from build123d import *

# Parameters (mm, degrees)
F0_R     = 9.525
F1_DEPTH = 6.35
F2_R     = 9.525
F3_DEPTH = 12.7


# Not quite as in the source:
# - a length typed as a fraction of an inch, garbled in the dataset ("3 / 203.2 mm" for 3/8 in), is restored


with BuildPart() as f1:
    # F0 (on Top) → F1 (new body)
    with BuildSketch(Plane.XY):
        with BuildLine():
            Line((12.7, 12.7), (0, 12.7))
            ThreePointArc((0, 12.7), (-12.7, 0), (0, -12.7))
            Line((0, -12.7), (12.7, -12.7))
            ThreePointArc((12.7, -12.7), (25.4, 0), (12.7, 12.7))
        make_face()
        Circle(F0_R, mode=Mode.SUBTRACT)
    extrude(amount=F1_DEPTH)

    # F2 (on face) → F3 (join)
    with BuildSketch(Plane(origin=(0, 0, 0), x_dir=(1, 0, 0), z_dir=(0, 0, -1))):
        with BuildLine():
            ThreePointArc((0, -12.7), (8.9802561211, -8.9802561211), (12.7, 0))
            ThreePointArc((12.7, 0), (8.9802561211, 8.9802561211), (0, 12.7))
            ThreePointArc((0, 12.7), (-12.7, 0), (0, -12.7))
        make_face()
        Circle(F2_R, mode=Mode.SUBTRACT)
    extrude(amount=F3_DEPTH)


solid = f1.part
Design review of the part built by this model. Coordinates are the model's own, in mm. A direction names the side the tool comes from. Coordinates: 2 decimals unless noted, no trailing zeros. Write each loop counter-clockwise with the first axis right and the second up, starting at its lowest first coordinate (ties: lowest second). Pieces come first, ordered by that corner, then holes. Notation, with made-up numbers: (-23, 75) - (-19, 75) arc R16 cw to (-19, 105) - close; hole circle Ø6 at (30, -11.5). An arc over 180 degrees is marked (long way). One line per item, written item: value.
1) Add section D-D (x = -0.5). State the section outline as (y, z) points.
Answer sheet:
outline: (-12.69, -12.7) - (-9.51, -12.7) - (-9.51, 6.35) - (-12.69, 6.35) - close; (9.51, -12.7) - (12.69, -12.7) - (12.69, 6.35) - (9.51, 6.35) - close
2) For faces 4 (the face through (10, 0, 6.35)), 5 (the face through (15, 0, 0)), list the 3-axis set-ups (+Z, -Z, +X, -X, +Y, -Y) from which the entire face can be reached by the end or side of a thin tool; tool diameter is ignored.
Answer sheet:
face 4: +Z, +X, -X, +Y, -Y
face 5: -Z, +X
3) Add section B-B (z = -5.75). State the section outline as (x, y) points (3 decimals).
Answer sheet:
outline: circle Ø25.4 at (0, 0); hole circle Ø19.05 at (0, 0)
4) Mouldability with a two-part tool opening along X and no side actions: class faces 1 (the face through (5, -9, -12.7)), 2 (the face through (-7.559, 5.796, -3.042)), 3 (the face through (25.397, -0.279, 3.131)) as +X half, -X half, draft (parallel to the pull), parting line (faces both ways), or undercut.
Answer sheet:
face 1: draft
face 2: undercut
face 3: +X half
5) To check wall thickness, follow probe 1 along Y at (x, z) = (0, 0.5) (3 decimals); probe 2 along X at (y, z) = (0, 2.75) (3 decimals). State the ranges of each line that lie inside material, in increasing order.
Answer sheet:
probe 1: y = -12.7 to -9.525, 9.525 to 12.7
probe 2: x = -12.7 to -9.525, 9.525 to 25.4
6) Add section A-A (x = 8). State the section outline as (y, z) points, plus the area to 3 significant figures.
Answer sheet:
outline: (-12.7, 0) - (-9.86, 0) - (-9.86, -12.7) - (-5.17, -12.7) - (-5.17, 6.35) - (-12.7, 6.35) - close; (5.17, -12.7) - (9.86, -12.7) - (9.86, 0) - (12.7, 0) - (12.7, 6.35) - (5.17, 6.35) - close
area: 215 mm2
7) Insertion check: pin 1 (8 mm diameter, centred on y = 7, z = -4.5, fed in from +X); pin 2 (8 mm diameter, centred on y = -6.5, z = -3.5, fed in from -X); pin 3 (12 mm diameter, centred on x = 7.5, y = -2, fed in from -Z); pin 4 (4 mm diameter, centred on y = 2, z = -2.5, fed in from +X). Each pin has a flat end and moves straight along its axis. Give the tip position at first contact, or say it passes through.
Answer sheet:
pin 1: stops at x = 12.34
pin 2: stops at x = -12.45
pin 3: stops at z = -12.7
pin 4: stops at x = 12.7
8) Add section C-C (y = -3). State the section outline as (x, z) points.
Answer sheet:
outline: (-12.34, -12.7) - (-9.04, -12.7) - (-9.04, 6.35) - (-12.34, 6.35) - close; (9.04, -12.7) - (12.34, -12.7) - (12.34, 0) - (25.04, 0) - (25.04, 6.35) - (9.04, 6.35) - close
